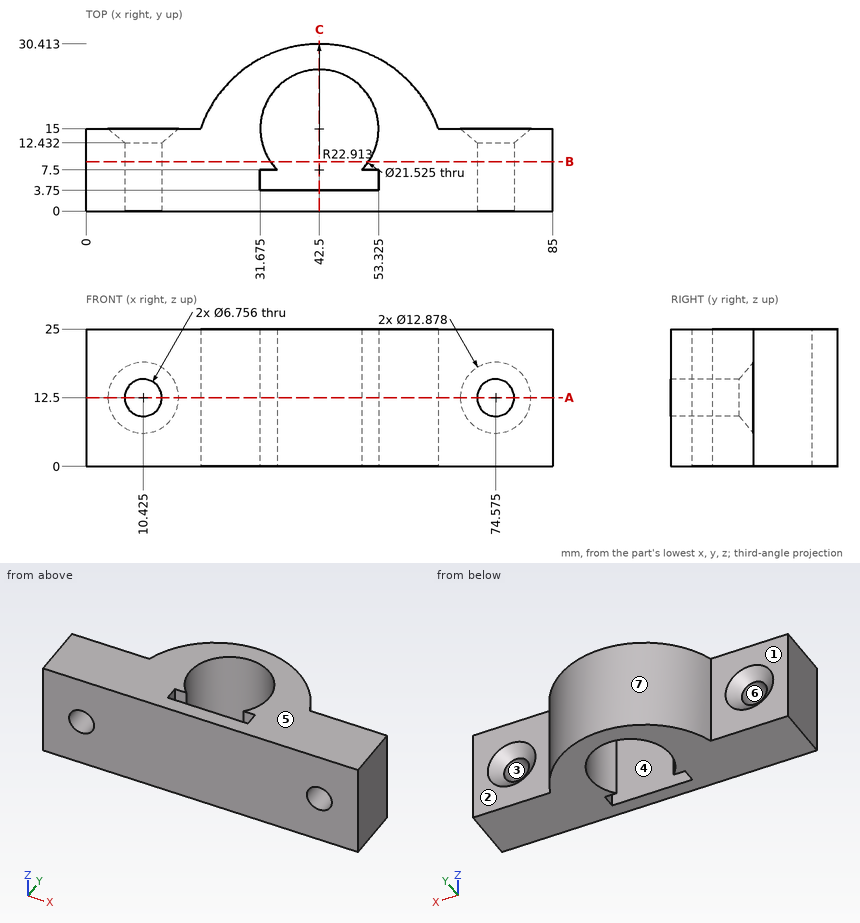
Geometry check sheet. Reference: drawing and pictorial views, mm from the part's lowest x, y, z. A direction names the side the tool comes from. Coordinates: 2 decimals unless noted, no trailing zeros. Write each loop counter-clockwise with the first axis right and the second up, starting at its lowest first coordinate (ties: lowest second). Pieces come first, ordered by that corner, then holes. Notation, with made-up numbers: (37, 70) - (93, 70) arc R14 cw to (93, 79) - close; hole circle Ø1 at (-6, 36). An arc over 180 degrees is marked (long way). Write item = value, one per line.
Q1. Cross-section at B-B (y = 9). Enter the section's corners in (x, z) (1 decimal), plus the area to 3 significant figures.
Answer:
outline = (0, 0) - (33.6, 0) - (33.6, 25) - (0, 25) - close; (51.4, 0) - (85, 0) - (85, 25) - (51.4, 25) - close; hole circle Ø6.8 at (10.4, 12.5); hole circle Ø6.8 at (74.6, 12.5)
area = 1,610 mm²
Q2. Cross-section at C-C (x = 42.5). Enter the section's corners in (y, z).
Answer:
outline = (0, 0) - (3.75, 0) - (3.75, 25) - (0, 25) - close; (25.76, 0) - (30.41, 0) - (30.41, 25) - (25.76, 25) - close
Q3. Material ranges on L1, parallel to X at y = 7.25, z = 12.5 (1 decimal); L2, parallel to X at y = 3.25, z = 12.5; L3, parallel to X at y = 9.75, z = 12.5 (1 decimal), recorded low to high. Write a range as from..to.
Answer:
L1 = 0..7, 13.8..31.7, 53.3..71.2, 78..85
L2 = 0..7.05, 13.8..71.2, 77.95..85
L3 = 0..7, 13.8..33.1, 51.9..71.2, 78..85
Q4. Access from +Z, -Z, +X, -X, +Y, -Y to the whole of each face (thin tool, end or side, straight path). Record for the marked faces 1, 2, 3 and 4.
Answer:
face_1 = +Z, -Z, -X, +Y
face_2 = +Z, -Z, +X, +Y
face_3 = +Y, -Y
face_4 = +Z, -Z
Q5. Go/stop test with flat-tipped pins: pin 1 Ø6 at (x, y) = (35, 14) entering from -Z; pin 2 Ø6.5 at (x, z) = (47.5, 9) entering from +Y; pin 3 Ø5 at (y, z) = (18, 7.5) entering from -X; pin 4 Ø4 at (y, z) = (19, 20.5) entering from +X. Record where each tip stops, or that it passes through.
Answer:
pin_1 = through
pin_2 = 30.35
pin_3 = 21.03
pin_4 = 63.35
Q6. Cross-section at A-A (z = 12.5). Give the number of separate pieces and of enclosed holes in the cut face, plus the area to 3 significant figures.
Answer:
separate_pieces = 3
enclosed_holes = 1
area = 1,130 mm²
Q7. Mould release check, pull along X, two halves, no side actions. Record for the marked faces 5, 6 and 7: released by +X, released by -X, zero draft, split by the parting line, or undercut.
Answer:
face_5 = zero draft
face_6 = undercut
face_7 = split by the parting line
